Design review of the part built by this model. Coordinates are the model's own, in mm. Face numbers are marked on the shaded views. A direction names the side the tool comes from. Round coordinates to 2 decimals unless told otherwise and drop trailing zeros. Loops run counter-clockwise (first coordinate to the right, second up) from the corner with the lowest first, then second, coordinate; pieces in that order, holes last. Notation, with made-up numbers: (11, 60) -> (21, 60) arc R16 cw to (21, 76) -> close; hole circle Ø3 at (18.5, 51). An arc over 180 degrees is marked (long way). Write each question's results on one line, items separated by ' | '. Start each with the question number.
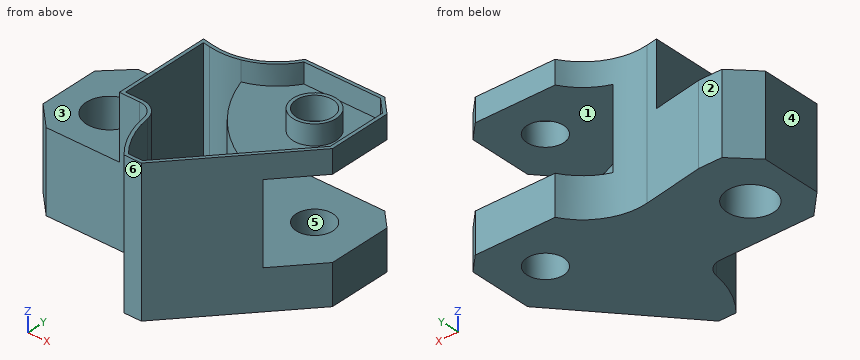
from build123d import *

# Parameters (mm, degrees)
SKETCH2_R               = 7
BOSS_EXTRUDE1_DEPTH     = 43
SKETCH3_R               = 5.5
CUT_EXTRUDE1_DEPTH      = 108.976849371
CUT_EXTRUDE2_DEPTH      = 108.976849371
CUT_EXTRUDE2_DEPTH_BACK = 19
SKETCH4_R               = 7
CUT_EXTRUDE12_START     = -24
CUT_EXTRUDE12_DEPTH     = 24
SHELL2_START            = 12
SHELL2_DEPTH            = 31
SHELL2_START_2          = 37
SHELL2_2_OUTLINE_R      = 6.5
SHELL2_2_DEPTH          = 6


# Read off the part's stored shape, not the designer's step: Shell2
with BuildPart() as part:
    # Sketch2 → Boss-Extrude1 (new body)
    with BuildSketch(Plane.XY):
        with BuildLine():
            Line((76, 57), (81, 52))
            Line((81, 52), (81, 33))
            Line((81, 33), (52, 0))
            Line((52, 0), (46.788067397, 0))
            ThreePointArc((46.788067397, 0), (42.3490952, 6.884327939), (40.012264997, 14.735294118))
            ThreePointArc((40.012264997, 14.735294118), (38.331862036, 17.786586232), (35.066626255, 19))
            Line((35.066626255, 19), (7, 19))
            Line((7, 19), (0, 26))
            Line((0, 26), (0, 44))
            Line((0, 44), (7, 51))
            Line((7, 51), (14, 51))
            Line((14, 51), (32.243084988, 47.783251905))
            ThreePointArc((32.243084988, 47.783251905), (43.574972961, 49.276069151), (52, 57))
            Line((52, 57), (76, 57))
        make_face()
        with Locations((14, 33)):
            Circle(SKETCH2_R, mode=Mode.SUBTRACT)
    extrude(amount=BOSS_EXTRUDE1_DEPTH)

    # Sketch3 → Cut-Extrude1 (cut, through all)
    with BuildSketch(Plane.XY.offset(43)):
        with Locations((67, 43)):
            Circle(SKETCH3_R)
    extrude(amount=-CUT_EXTRUDE1_DEPTH, mode=Mode.SUBTRACT)

    # Sketch4 → Cut-Extrude2 (cut, two sides: drawn at the far end of the back side and taken through both)
    with BuildSketch(Plane.XY.offset(43).offset(-CUT_EXTRUDE2_DEPTH_BACK)):
        Polygon((29, 19), (29, 48.355095289), (14, 51), (7, 51), (0, 44), (0, 26), (7, 19), align=None)
        with Locations((14, 33)):
            Circle(SKETCH4_R, mode=Mode.SUBTRACT)
    extrude(amount=CUT_EXTRUDE2_DEPTH + CUT_EXTRUDE2_DEPTH_BACK, mode=Mode.SUBTRACT)

    # Sketch7 → Cut-Extrude12 (cut)
    with BuildSketch(Plane.XY.offset(36).offset(CUT_EXTRUDE12_START)):
        with BuildLine():
            ThreePointArc((52, 57), (47.665353397, 51.864697991), (41.814145925, 48.559571819))
            ThreePointArc((41.814145925, 48.559571819), (52.571435773, 31.077146254), (70.454545455, 21))
            Line((70.454545455, 21), (81, 33))
            Line((81, 33), (81, 52))
            Line((81, 52), (76, 57))
            Line((76, 57), (52, 57))
        make_face()
    extrude(amount=CUT_EXTRUDE12_DEPTH, mode=Mode.SUBTRACT)

    # Shell2 outline → Shell2 (cut)
    with BuildSketch(Plane.XY.offset(SHELL2_START)):
        with BuildLine():
            Line((51.547522264, 1), (68.661045623, 20.47400934))
            ThreePointArc((68.661045623, 20.47400934), (51.667497173, 30.560606948), (41.16767498, 47.301989033))
            ThreePointArc((41.16767498, 47.301989033), (36.647615315, 46.525160064), (32.06943681, 46.798444152))
            Line((32.06943681, 46.798444152), (30, 47.163341697))
            Line((30, 47.163341697), (30, 20))
            Line((30, 20), (35.066626255, 20))
            ThreePointArc((35.066626255, 20), (38.984909193, 18.543903479), (41.001392745, 14.882352941))
            ThreePointArc((41.001392745, 14.882352941), (43.163792236, 7.508400948), (47.249359107, 1))
            Line((47.249359107, 1), (51.547522264, 1))
        make_face()
    extrude(amount=SHELL2_DEPTH, mode=Mode.SUBTRACT)

    # Shell2 2 outline → Shell2 2 (cut)
    with BuildSketch(Plane.XY.offset(SHELL2_START_2)):
        with BuildLine():
            Line((68.661045623, 20.47400934), (80, 33.376957423))
            Line((80, 33.376957423), (80, 51.585786438))
            Line((80, 51.585786438), (75.585786438, 56))
            Line((75.585786438, 56), (52.567775172, 56))
            ThreePointArc((52.567775172, 56), (47.674046111, 50.594185021), (41.16767498, 47.301989034))
            ThreePointArc((41.16767498, 47.301989034), (51.667497173, 30.560606948), (68.661045623, 20.47400934))
        make_face()
        with Locations((67, 43)):
            Circle(SHELL2_2_OUTLINE_R, mode=Mode.SUBTRACT)
    extrude(amount=SHELL2_2_DEPTH, mode=Mode.SUBTRACT)


solid = part.part
1) Take a section at B-B (z = 7). Write out the cut boundary in (x, y).
2) Take a section at A-A (x = 67). Write out the cut boundary in (y, z).
3) For the marked faces 1, 2 and 3, list the 3-axis set-ups (+Z, -Z, +X, -X, +Y, -Y) from which the entire face can be reached by the end or side of a thin tool; tool diameter is ignored.
4) Take a section at D-D (y = 23). Write out the cut boundary in (x, z).
5) Insertion check: pin 1 (1 mm diameter, centred on x = 50, y = 46.5, fed in from +Z); pin 2 (6 mm diameter, centred on y = 12, z = 35, fed in from -X); pin 3 (15 mm diameter, centred on y = 40.5, z = 37, fed in from -X). Each pin has a flat end and moves straight along its axis. Give the tip position at first contact, or say it passes through.
6) To check wall thickness, follow line 1 (Y direction, x = 14, z = 12.5); line 2 (X direction, y = 34.5, z = 13); line 3 (Y direction, x = 63.5, z = 37.5). State the ranges of each line that lie inside material, in increasing order. Write a range as from..to.
7) Take a section at C-C (z = 31). Write out the cut boundary in (x, y).
8) The part is to be moulded in two halves that separate along X. For the marked faces 4, 5 and 6, say which applies: +X half, -X half, draft (parallel to the pull), parting line (faces both ways), or undercut.
Geometry check:
1) outline: (0, 26) -> (7, 19) -> (35.07, 19) arc R5 cw to (40.01, 14.74) arc R29 ccw to (46.79, 0) -> (52, 0) -> (81, 33) -> (81, 52) -> (76, 57) -> (52, 57) arc R19 cw to (32.24, 47.78) -> (14, 51) -> (7, 51) -> (0, 44) -> close; hole circle Ø14 at (14, 33); hole circle Ø11 at (67, 43)
2) outline: (17.07, 0) -> (37.5, 0) -> (37.5, 12) -> (22.08, 12) -> (22.08, 36) -> (37.5, 36) -> (37.5, 43) -> (36.5, 43) -> (36.5, 37) -> (21.02, 37) -> (21.02, 12) -> (18.58, 12) -> (18.58, 43) -> (17.07, 43) -> close; (48.5, 0) -> (57, 0) -> (57, 12) -> (48.5, 12) -> close; (48.5, 36) -> (57, 36) -> (57, 43) -> (56, 43) -> (56, 37) -> (49.5, 37) -> (49.5, 43) -> (48.5, 43) -> close
3) face 1: +X, +Y | face 2: +Z, -Z, -X, +Y | face 3: +Z, -X, +Y, -Y
4) outline: (3, 0) -> (72.21, 0) -> (72.21, 12) -> (64.7, 12) -> (64.7, 36) -> (72.21, 36) -> (72.21, 43) -> (70.88, 43) -> (70.88, 37) -> (62.33, 37) -> (62.33, 12) -> (30, 12) -> (30, 43) -> (29, 43) -> (29, 24) -> (3, 24) -> close
5) pin 1: stops at z = 37 | pin 2: stops at x = 39.97 | pin 3: stops at x = 29
6) line 1: y = 19..26, 40..51 | line 2: x = 0..7.16, 20.84..30, 48.11..49.4 | line 3: y = 13.09..14.6, 37.52..38.76, 47.24..48.48, 56..57
7) outline: (29, 19) -> (35.07, 19) arc R5 cw to (40.01, 14.74) arc R29 ccw to (46.79, 0) -> (52, 0) -> (70.45, 21) arc R41 cw to (41.81, 48.56) arc R19 cw to (32.24, 47.78) -> (29, 48.36) -> close; hole (30, 20) -> (35.07, 20) arc R6 cw to (41, 14.88) arc R28 ccw to (47.25, 1) -> (51.55, 1) -> (68.66, 20.47) arc R42 cw to (41.17, 47.3) arc R20 cw to (32.07, 46.8) -> (30, 47.16) -> close
8) face 4: -X half | face 5: undercut | face 6: draft
